The figure shows three views and two pictorial views of one solid part (mm, origin at its lowest corner). Answer the questions. Round coordinates to 2 decimals unless told otherwise and drop trailing zeros. Order: outer loops, then holes, each group sorted by start corner. A loop starts at its lowest first (then second) coordinate and runs counter-clockwise, first axis right, second up. Notation, with made-up numbers: (32, 45) -> (85, 45) arc R25 ccw to (85, 64) -> close; hole circle Ø11 at (-4, 80.5). An arc over 180 degrees is marked (long way). One line per item, written item: value. Start each with the question number.
1. Section B-B (z = 40) is taken. Give the vertices of the cut face in (x, y), then the cut area to 3 significant figures.
2. A flat-ended cylindrical pin translates along its axis: pin 1 Ø4 at (x, z) = (16.5, 37.5) entering from -Y. Find the tip coordinate at first contact, or state that the pin passes through.
3. Section A-A (x = 10) is taken. Give the vertices of the cut face in (y, z), then the cut area to 3 significant figures.
4. Section D-D (z = 70) is taken. Give the vertices of the cut face in (x, y), then the cut area to 3 significant figures.
5. Section C-C (x = 40) is taken. Give the vertices of the cut face in (y, z), then the cut area to 3 significant figures.
6. Consider line 1 (X direction, y = 7, z = 70); line 2 (Z direction, x = 40, y = 3.25). Determine where each line is inside the solid, lowest interval first.
7. The mould has two halves that part along Z. Classify the marked faces 1, 2, 3 and 4: released by +Z, released by -Z, zero draft, split by the parting line, or undercut.
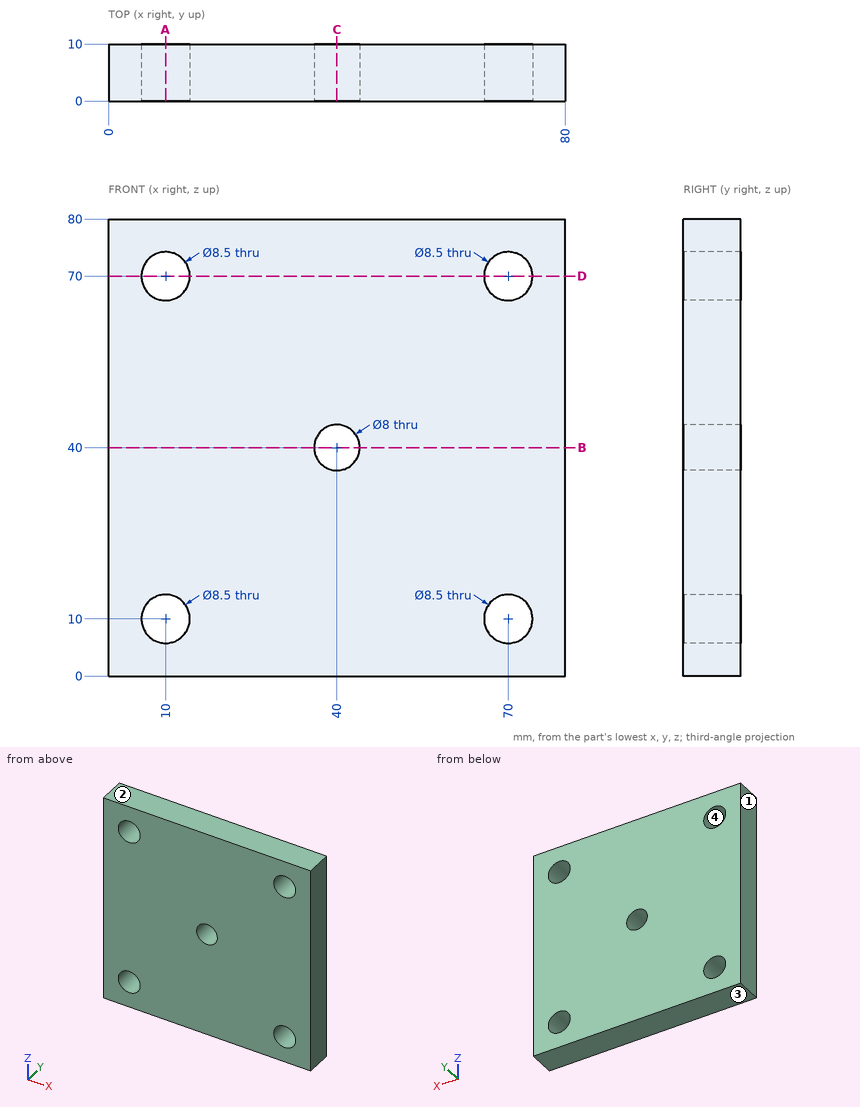
Answer:
1. outline: (0, 0) -> (36, 0) -> (36, 10) -> (0, 10) -> close; (44, 0) -> (80, 0) -> (80, 10) -> (44, 10) -> close
1. area: 720 mm^2
2. pin 1: y = 0
3. outline: (0, 0) -> (10, 0) -> (10, 5.75) -> (0, 5.75) -> close; (0, 14.25) -> (10, 14.25) -> (10, 65.75) -> (0, 65.75) -> close; (0, 74.25) -> (10, 74.25) -> (10, 80) -> (0, 80) -> close
3. area: 630 mm^2
4. outline: (0, 0) -> (5.75, 0) -> (5.75, 10) -> (0, 10) -> close; (14.25, 0) -> (65.75, 0) -> (65.75, 10) -> (14.25, 10) -> close; (74.25, 0) -> (80, 0) -> (80, 10) -> (74.25, 10) -> close
4. area: 630 mm^2
5. outline: (0, 0) -> (10, 0) -> (10, 36) -> (0, 36) -> close; (0, 44) -> (10, 44) -> (10, 80) -> (0, 80) -> close
5. area: 720 mm^2
6. line 1: 0 to 5.75, 14.25 to 65.75, 74.25 to 80
6. line 2: 0 to 36, 44 to 80
7. face 1: zero draft
7. face 2: released by +Z
7. face 3: released by -Z
7. face 4: undercut
